Geometry: final body of the model. Coordinates: model frame, mm. Face numbers are marked on the shaded views. A direction names the side the tool comes from. Round coordinates to 2 decimals unless told otherwise and drop trailing zeros. Order: outer loops, then holes, each group sorted by start corner. A loop starts at its lowest first (then second) coordinate and runs counter-clockwise, first axis right, second up. Notation, with made-up numbers: (28.25, 48.5) -> (49.25, 48.5) arc R13 ccw to (49.25, 56.5) -> close; hole circle Ø9 at (61.5, 29.25). An arc over 180 degrees is marked (long way). Put each result on its own line as item: value.
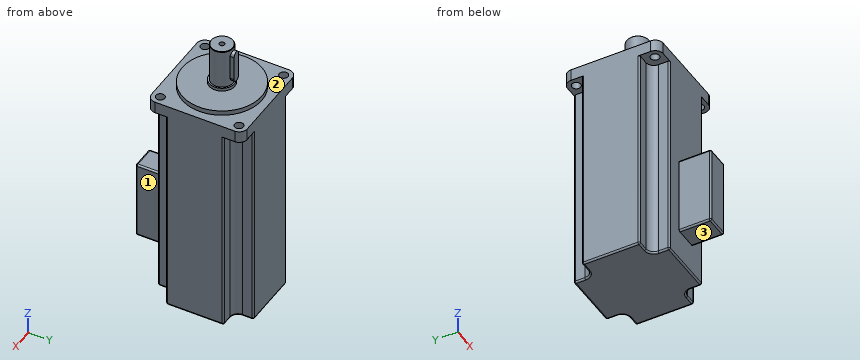
```python
from build123d import *

# Parameters (mm, degrees)
SKETCH_1_W             = 60.2
SKETCH_1_H             = 60.2
EXTRUDE_1_DEPTH        = 7.5
FILLET_1_R             = 5
SKETCH_2_R             = 2.75
CUT_EXTRUDE_1_DEPTH    = 44.223488985
SKETCH_3_R             = 25
EXTRUDE_2_DEPTH        = 3
SKETCH_4_R             = 8
EXTRUDE_3_DEPTH        = 2
SKETCH_5_R             = 7
EXTRUDE_4_DEPTH        = 25
HOLE_WIZARD_M4_2_D     = 3.3
HOLE_WIZARD_M4_2_DEPTH = 10.1
HOLE_WIZARD_M4_2_TIP   = 0.991420021
CHAMFER_1_SIZE         = 0.3
EXTRUDE_5_DEPTH        = 5
EXTRUDE_6_DEPTH        = 133.5
FILLET_2_R             = 5
SKETCH_13_W            = 15
SKETCH_13_H            = 50
EXTRUDE_7_DEPTH        = 20
FILLET_3_R             = 1


with BuildPart() as part:
    # 草图1 → 凸台-拉伸1 (new body)
    with BuildSketch(Plane.XY):
        Rectangle(SKETCH_1_W, SKETCH_1_H)
    extrude(amount=EXTRUDE_1_DEPTH)

    # 圆角1
    fillet_1_edges = [part.edges().sort_by_distance(p)[0] for p in [
        (30.1, -30.1, 3.75),
        (-30.1, -30.1, 3.75),
        (-30.1, 30.1, 3.75),
        (30.1, 30.1, 3.75),
    ]]
    fillet(fillet_1_edges, radius=FILLET_1_R)

    # 草图2 → 切除-拉伸1 (cut, through all)
    with BuildSketch(Plane.XY.offset(7.5)):
        with Locations((-24.748737342, 24.748737342)):
            Circle(SKETCH_2_R)
        with Locations((24.748737342, 24.748737342)):
            Circle(SKETCH_2_R)
        with Locations((24.748737342, -24.748737342)):
            Circle(SKETCH_2_R)
        with Locations((-24.748737342, -24.748737342)):
            Circle(SKETCH_2_R)
    extrude(amount=-CUT_EXTRUDE_1_DEPTH, mode=Mode.SUBTRACT)

    # 草图3 → 凸台-拉伸2 (add)
    with BuildSketch(Plane.XY.offset(7.5)):
        with Locations(Location((0, 0, 0), (0, 0, 180))):
            Circle(SKETCH_3_R)
    extrude(amount=EXTRUDE_2_DEPTH)

    # 草图4 → 凸台-拉伸3 (add)
    with BuildSketch(Plane.XY.offset(10.5)):
        Circle(SKETCH_4_R)
    extrude(amount=EXTRUDE_3_DEPTH)

    # 草图5 → 凸台-拉伸4 (add)
    with BuildSketch(Plane.XY.offset(12.5)):
        Circle(SKETCH_5_R)
    extrude(amount=EXTRUDE_4_DEPTH)

    # M4 螺纹孔2
    with Locations(Plane.XY.offset(37.5)):
        with Locations((0, 0)):
            Hole(HOLE_WIZARD_M4_2_D / 2, depth=HOLE_WIZARD_M4_2_DEPTH)
            with Locations((0, 0, -(HOLE_WIZARD_M4_2_DEPTH + HOLE_WIZARD_M4_2_TIP / 2))):  # 118° drill point
                Cone(0, HOLE_WIZARD_M4_2_D / 2, HOLE_WIZARD_M4_2_TIP, mode=Mode.SUBTRACT)

    # 倒角1
    chamfer_1_edges = [part.edges().sort_by_distance(p)[0] for p in [
        (-7, 0, 37.5),
    ]]
    chamfer(chamfer_1_edges, length=CHAMFER_1_SIZE)

    # 草图10 → 凸台-拉伸5 (add)
    with BuildSketch(Plane(origin=(0, 9, 0), x_dir=(1, 0, 0), z_dir=(0, 1, 0))):
        with BuildLine():
            Line((-2.5, -33), (-2.5, -17.5))
            ThreePointArc((-2.5, -17.5), (0, -15), (2.5, -17.5))
            Line((2.5, -17.5), (2.5, -33))
            ThreePointArc((2.5, -33), (0, -35.5), (-2.5, -33))
        make_face()
    extrude(amount=-EXTRUDE_5_DEPTH)

    # 草图12 → 凸台-拉伸6 (add)
    with BuildSketch(Plane(origin=(0, 0, 0), x_dir=(-1, 0, 0), z_dir=(0, 0, -1))):
        Polygon((30.1, -18.1), (18.1, -18.1), (18.1, -30.1), (-18.1, -30.1), (-18.1, -18.1), (-30.1, -18.1), (-30.1, 18.1), (-18.1, 18.1), (-18.1, 30.1), (18.1, 30.1), (18.1, 18.1), (30.1, 18.1), align=None)
    extrude(amount=EXTRUDE_6_DEPTH)

    # 圆角2
    fillet_2_edges = [part.edges().sort_by_distance(p)[0] for p in [
        (-18.1, 18.1, -66.75),
        (18.1, 18.1, -66.75),
        (18.1, -18.1, -66.75),
        (-18.1, -18.1, -66.75),
    ]]
    fillet(fillet_2_edges, radius=FILLET_2_R)

    # 草图13 → 凸台-拉伸7 (add)
    with BuildSketch(Plane.XZ.offset(30.1)):
        with Locations((0, -88.5)):
            Rectangle(SKETCH_13_W, SKETCH_13_H)
    extrude(amount=EXTRUDE_7_DEPTH)

    # 圆角3
    fillet_3_edges = [part.edges().sort_by_distance(p)[0] for p in [
        (-30.1, -18.1, -66.75),
        (-30.1, 18.1, -66.75),
        (-18.1, 30.1, -66.75),
        (18.1, 30.1, -66.75),
        (30.1, 18.1, -66.75),
        (30.1, -18.1, -66.75),
        (18.1, -30.1, -66.75),
        (-18.1, -30.1, -66.75),
        (-30.1, 0, -133.5),
        (-26.6, 18.1, -133.5),
        (0, 30.1, -133.5),
        (18.1, 26.6, -133.5),
        (30.1, 0, -133.5),
        (26.6, -18.1, -133.5),
        (0, -30.1, -133.5),
        (-18.1, -26.6, -133.5),
        (-26.6, -18.1, -133.5),
        (-18.1, 26.6, -133.5),
        (26.6, 18.1, -133.5),
        (18.1, -26.6, -133.5),
        (-19.564466094, -19.564466094, -133.5),
        (-19.564466094, 19.564466094, -133.5),
        (19.564466094, 19.564466094, -133.5),
        (19.564466094, -19.564466094, -133.5),
        (-7.5, -40.1, -63.5),
        (-7.5, -40.1, -113.5),
        (7.5, -40.1, -113.5),
        (7.5, -40.1, -63.5),
        (-7.5, -50.1, -88.5),
        (0, -50.1, -113.5),
        (7.5, -50.1, -88.5),
        (0, -50.1, -63.5),
    ]]
    fillet(fillet_3_edges, radius=FILLET_3_R)


solid = part.part
```
1. Material intervals for probe 1 along Y at (x, z) = (0, 32.25); probe 2 along Z at (x, y) = (21, -9.5); probe 3 along X at (y, z) = (26, -4), sorted ascending.
Ans:
probe 1: -7 to -1.65, 1.65 to 9
probe 2: -133.5 to 10.5
probe 3: -18.1 to 18.1
2. Set-up query: the marked faces 1, 2 and 3. Return all of +Z, -Z, +X, -X, +Y, -Y with unobstructed straight access to the full face (end or side cutting, diameter ignored); none if empty.
Ans:
face 1: +Z, -Z, +X, -Y
face 2: +Z
face 3: -Z, +X, -X, -Y
3. Cut plane B-B on x = -11.5. Return loops of the section in (y, z).
Ans:
outline: (-30.1, -132.5) arc R1 ccw to (-29.1, -133.5) -> (29.1, -133.5) arc R1 ccw to (30.1, -132.5) -> (30.1, 7.5) -> (22.2, 7.5) -> (22.2, 10.5) -> (-22.2, 10.5) -> (-22.2, 7.5) -> (-30.1, 7.5) -> close
4. Contact query for flat-ended pins moving along their axis: P1, Ø14.5, axis at x = 26.5, y = 23, coming from the -Z side; P2, Ø14.5, axis at x = -26.5, y = -25, coming from the -Z side; P3, Ø1.5, axis at x = 22, z = -30, coming from the -Y side; P4, Ø10.5, axis at x = -1, y = -44, coming from the +Z side. Output: stop coordinate, or through.
Ans:
P1: z = -133.5
P2: z = -133.26
P3: y = -18.45
P4: z = -63.5
5. Cut plane A-A on z = -51.5. Return loops of the section in (x, y).
Ans:
outline: (-30.1, -17.1) arc R1 ccw to (-29.1, -18.1) -> (-23.1, -18.1) arc R5 cw to (-18.1, -23.1) -> (-18.1, -29.1) arc R1 ccw to (-17.1, -30.1) -> (17.1, -30.1) arc R1 ccw to (18.1, -29.1) -> (18.1, -23.1) arc R5 cw to (23.1, -18.1) -> (29.1, -18.1) arc R1 ccw to (30.1, -17.1) -> (30.1, 17.1) arc R1 ccw to (29.1, 18.1) -> (23.1, 18.1) arc R5 cw to (18.1, 23.1) -> (18.1, 29.1) arc R1 ccw to (17.1, 30.1) -> (-17.1, 30.1) arc R1 ccw to (-18.1, 29.1) -> (-18.1, 23.1) arc R5 cw to (-23.1, 18.1) -> (-29.1, 18.1) arc R1 ccw to (-30.1, 17.1) -> close
